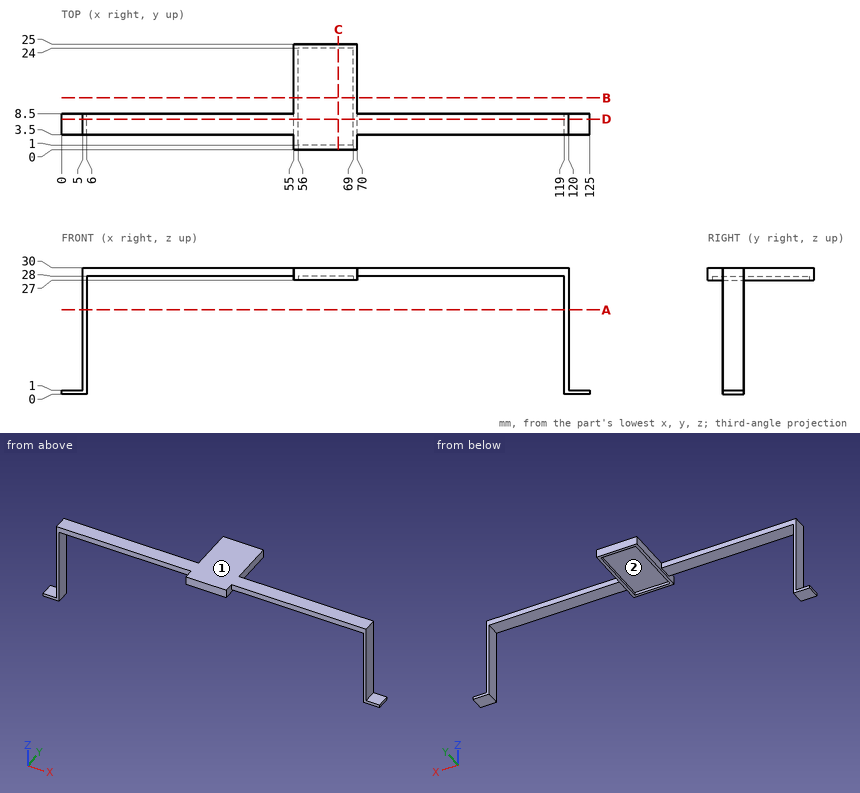
Job drawing, mm, ordinate dimensions from the low corner. One solid piece. Give positions to 0.01 mm unless a question says otherwise; leave off trailing zeros. Order: outer loops, then holes, each group sorted by start corner. A loop starts at its lowest first (then second) coordinate and runs counter-clockwise, first axis right, second up. Notation, with made-up numbers: (60, 6.5) - (70, 6.5) arc R6 ccw to (70, 10.5) - close; hole circle Ø6 at (19.25, -10.5). An arc over 180 degrees is marked (long way). Return JSON: item names as keys, results as strings.
1) Cut at C-C, the plane x = 65.5. Give the cut face in (y, z).
Geometry says:
{"outline": "(0, 27) - (1, 27) - (1, 28) - (24, 28) - (24, 27) - (25, 27) - (25, 30) - (0, 30) - close"}
2) Cut at B-B, the plane y = 12.25. Give the cut face in (x, z), plus the area to 3 significant figures.
Geometry says:
{"outline": "(55, 27) - (56, 27) - (56, 28) - (69, 28) - (69, 27) - (70, 27) - (70, 30) - (55, 30) - close", "area": "32.0 mm²"}
3) Cut at A-A, the plane z = 20. Give the cut face in (x, y).
Geometry says:
{"outline": "(5, 3.5) - (6, 3.5) - (6, 8.5) - (5, 8.5) - close; (119, 3.5) - (120, 3.5) - (120, 8.5) - (119, 8.5) - close"}
4) Probe line 1 (X direction, y = 4.25, z = 19); line 2 (Z direction, x = 20, y = 5); line 3 (X direction, y = 23.5, z = 27.25). List the from-to ranges inside material, lowest first. Write a range as from..to.
Geometry says:
{"line 1": "5..6, 119..120", "line 2": "28..30", "line 3": "55..56, 69..70"}
5) Cut at D-D, the plane y = 7.25. Give the cut face in (x, z), plus the area to 3 significant figures.
Geometry says:
{"outline": "(0, 0) - (6, 0) - (6, 28) - (55, 28) - (55, 27) - (56, 27) - (56, 28) - (69, 28) - (69, 27) - (70, 27) - (70, 28) - (119, 28) - (119, 0) - (125, 0) - (125, 1) - (120, 1) - (120, 30) - (5, 30) - (5, 1) - (0, 1) - close", "area": "298 mm²"}
6) Pull direction Y, two halves, no side cores. Call the marked faces 1 and 2: pulls with the +Y half, pulls with the -Y half, needs draft (parallel to the pull), parting line crosses it, or undercut.
Geometry says:
{"face 1": "needs draft", "face 2": "undercut"}
7) Flat gauge pins, fed straight in: P1, Ø12, axis at x = 28.5, y = 8, coming from the -Z side; P2, Ø5.5, axis at x = 2, y = 5, coming from the +Z side; P3, Ø4, axis at y = 6.5, z = 13.5, coming from the -X side. Where does each tip first touch, or does it go through?
Geometry says:
{"P1": "z = 28", "P2": "z = 1", "P3": "x = 5"}
